Could you check a few things on this drawing? It's one solid part, dimensions in mm from its lowest x, y, z. A direction names the side the tool comes from. Round coordinates to 2 decimals unless told otherwise and drop trailing zeros. Loops run counter-clockwise (first coordinate to the right, second up) from the corner with the lowest first, then second, coordinate; pieces in that order, holes last. Notation, with made-up numbers: M 41.5,22 L 85.5,22 A16 ccw 85.5,44 Z; hole C 71.5,76 d11. An arc over 180 degrees is marked long. Return JSON: item names as keys, results as strings.
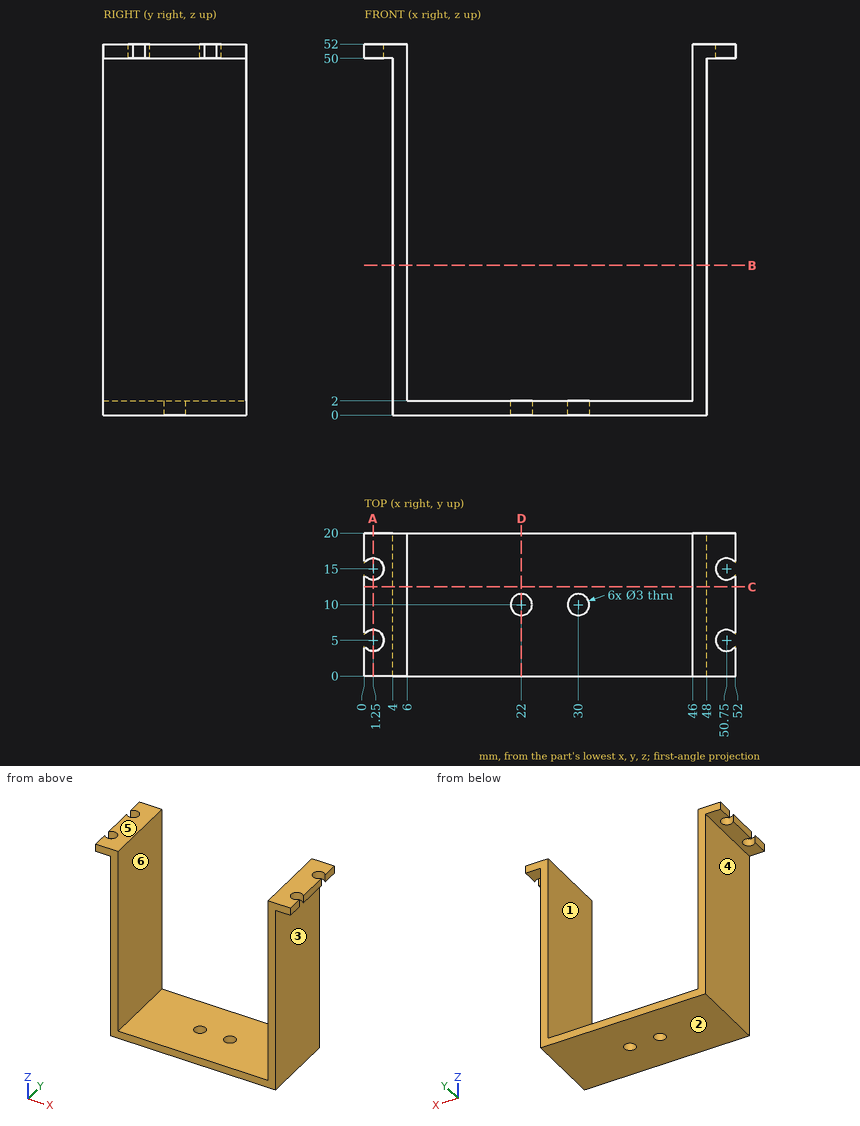
Q1. I'm going to push flat-ended pins straight in: pin 1 Ø10 at (y, z) = (11.5, 25) entering from -X; pin 2 Ø1 at (x, y) = (10.5, 8) entering from +Z; pin 3 Ø5 at (x, y) = (50.75, 15) entering from -Z. Where does each tip first touch, or does it pass through?
Results:
{"pin 1": "stops at x = 4", "pin 2": "stops at z = 2", "pin 3": "stops at z = 50"}
Q2. Suppose I cut it at A-A, the plane x = 1.25. Please give me the cut outline in (y, z), plus the area to 3 significant figures.
Results:
{"outline": "M 0,50 L 3.5,50 L 3.5,52 L 0,52 Z; M 6.5,50 L 13.5,50 L 13.5,52 L 6.5,52 Z; M 16.5,50 L 20,50 L 20,52 L 16.5,52 Z", "area": "28.0 mm2"}
Q3. Suppose I cut it at C-C, the plane y = 12.5. Please give me the cut outline in (x, z), plus the area to 3 significant figures.
Results:
{"outline": "M 0,50 L 4,50 L 4,0 L 48,0 L 48,50 L 52,50 L 52,52 L 46,52 L 46,2 L 6,2 L 6,52 L 0,52 Z", "area": "304 mm2"}
Q4. Thinking about a two-plate mould opening in X: for the marked faces 1, 2 and 3, which applies, pulls with the +X half, pulls with the -X half, needs draft (parallel to the pull), parting line crosses it, or undercut?
Results:
{"face 1": "undercut", "face 2": "needs draft", "face 3": "pulls with the +X half"}
Q5. Suppose I cut it at D-D, the plane x = 22. Please give me the cut outline in (y, z), plus the area to 3 significant figures.
Results:
{"outline": "M 0,0 L 8.5,0 L 8.5,2 L 0,2 Z; M 11.5,0 L 20,0 L 20,2 L 11.5,2 Z", "area": "34.0 mm2"}
Q6. Suppose I cut it at B-B, the plane z = 21. Please give me the cut outline in (x, y).
Results:
{"outline": "M 4,0 L 6,0 L 6,20 L 4,20 Z; M 46,0 L 48,0 L 48,20 L 46,20 Z"}
Q7. On a 3-axis mill with a long thin cutter (end or side, diameter ignored), from which of +Z, -Z, +X, -X, +Y, -Y can I reach the whole of each face in a straight line? I mean the marked faces 4, 5 and 6. Say none if no direction works.
Results:
{"face 4": "-Z, -X, +Y, -Y", "face 5": "+Z, +X, -X, +Y, -Y", "face 6": "+Z, +Y, -Y"}
Q8. If I drill on line 1 along X through (y, z) = (1.75, 49.5); line 2 along Y through (x, z) = (1.25, 51.5); line 3 along X through (y, z) = (15, 50.5), over which ranges is the centre line in solid material (lowest first)?
Results:
{"line 1": "x = 4 to 6, 46 to 48", "line 2": "y = 0 to 3.5, 6.5 to 13.5, 16.5 to 20", "line 3": "x = 2.75 to 6, 46 to 49.25"}
